Verification items for the finished model (mm, model axes). A direction names the side the tool comes from. Give positions to 0.01 mm unless a question says otherwise; leave off trailing zeros. Loops run counter-clockwise (first coordinate to the right, second up) from the corner with the lowest first, then second, coordinate; pieces in that order, holes last. Notation, with made-up numbers: M 23.25,35.25 L 37.25,35.25 A34 cw 37.25,70.25 Z; hole C -7.5,27.5 d2. An arc over 180 degrees is marked long. Use CSV: the item, a comma, the result in double quotes.
from build123d import *

# Parameters (mm, degrees)
F0_W        = 30
F0_H        = 5
F1_DEPTH    = 2
F2_R        = 5
F3_T1_DEPTH = 27


# Not quite as in the source:
# - a fillet or chamfer that OpenCascade refuses, or shapes differently, is made with other operations: its cross-section is extruded or revolved along the edge and cut away or added
# - a feature names something its author has since deleted; it is built from what else it names


with BuildPart() as f1:
    # F0 (on Top) → F1 (new body)
    with BuildSketch(Plane.XY):
        Polygon((0, 15), (0, 10), (30, 10), (30, 15), (8, 15), (4, 15), align=None)
        with Locations((15, 2.5)):
            Rectangle(F0_W, F0_H)
        with BuildLine():
            Line((0, 7.5), (0, 5))
            Line((0, 5), (30, 5))
            Line((30, 5), (30, 7.5))
            Line((30, 7.5), (24, 7.5))
            ThreePointArc((24, 7.5), (22.5, 6), (21, 7.5))
            Line((21, 7.5), (15, 7.5))
            Line((15, 7.5), (9, 7.5))
            ThreePointArc((9, 7.5), (7.5, 6), (6, 7.5))
            Line((6, 7.5), (0, 7.5))
        make_face()
        with BuildLine():
            Line((0, 10), (0, 7.5))
            Line((0, 7.5), (6, 7.5))
            ThreePointArc((6, 7.5), (7.5, 9), (9, 7.5))
            Line((9, 7.5), (15, 7.5))
            Line((15, 7.5), (21, 7.5))
            ThreePointArc((21, 7.5), (22.5, 9), (24, 7.5))
            Line((24, 7.5), (30, 7.5))
            Line((30, 7.5), (30, 10))
            Line((30, 10), (0, 10))
        make_face()
        Polygon((0, 60), (0, 15), (4, 15), (8, 15), (8, 60), align=None)
        Polygon((5, 25), (4, 25), (3, 25), (3, 55), (5, 55), align=None, mode=Mode.SUBTRACT)
    extrude(amount=F1_DEPTH)

    # F2
    f2_edges = [f1.edges().sort_by_distance(p)[0] for p in [
        (8, 15, 1),
        (30, 15, 1),
        (30, 0, 1),
        (0, 0, 1),
    ]]
    fillet(f2_edges, radius=F2_R)

    # F3: fillet of radius 5 on 2 edges, made by hand

    # F3_s2 → F3_t1 (cut)
    with BuildSketch(Plane.XY.offset(-12.5)):
        with BuildLine():
            ThreePointArc((3, 60), (6.5355339059, 58.5355339059), (8, 55))
            Line((8, 55), (8, 60))
            Line((8, 60), (3, 60))
        make_face()
        with BuildLine():
            ThreePointArc((0, 55), (1.4644660941, 58.5355339059), (5, 60))
            Line((5, 60), (0, 60))
            Line((0, 60), (0, 55))
        make_face()
    extrude(amount=F3_T1_DEPTH, mode=Mode.SUBTRACT)


solid = f1.part
(1) Section check A-A on x = 22.5. Record the cut outline in (y, z), plus the area to 3 significant figures.
Calculated:
outline,"M 0,0 L 6,0 L 6,2 L 0,2 Z; M 9,0 L 15,0 L 15,2 L 9,2 Z"
area,"24.0 mm²"
(2) Section check B-B on y = 7.5. Record the cut outline in (x, z).
Calculated:
outline,"M 0,0 L 6,0 L 6,2 L 0,2 Z; M 9,0 L 21,0 L 21,2 L 9,2 Z; M 24,0 L 30,0 L 30,2 L 24,2 Z"
(3) Section check D-D on z = 1.6. Record the cut outline in (x, y), plus the area to 3 significant figures.
Calculated:
outline,"M 0,5 A5 ccw 5,0 L 25,0 A5 ccw 30,5 L 30,10 A5 ccw 25,15 L 13,15 A5 cw 8,20 L 8,55 A5 ccw 4,59.9 A5 ccw 0,55 Z; hole M 3,25 L 5,25 L 5,55 L 3,55 Z; hole C 7.5,7.5 d3; hole C 22.5,7.5 d3"
area,"714 mm²"
(4) Depth check by flat-ended pin: pin 1 Ø1 at (x, z) = (22.5, 1.5) entering from +Y; pin 2 Ø0.6 at (y, z) = (30, 0.5) entering from +X. Enter the tip coordinate at first touch or a pass-through.
Calculated:
pin 1,"stops at y = 15"
pin 2,"stops at x = 8"
(5) Tool access check on faces 1 (the flat face through (4, 55, 1)), 2 (the flat face through (15, 0, 1)), 3 (the flat face through (8, 37, 1)). Record the directions out of +Z, -Z, +X, -X, +Y, -Y that give a thin tool (end or side, any length) a straight path to the whole face; none if there is none.
Calculated:
face 1,"+Z, -Z"
face 2,"+Z, -Z, +X, -X, -Y"
face 3,"+Z, -Z, +X, +Y"
(6) Scan lines: L1, parallel to X at y = 7.5, z = 0.5; L2, parallel to X at y = 35, z = 1.7; L3, parallel to Y at x = 22.5, z = 1.15. Record each from-to range of solid material in increasing order. Write a range as from..to.
Calculated:
L1,"x = 0..6, 9..21, 24..30"
L2,"x = 0..3, 5..8"
L3,"y = 0..6, 9..15"
(7) Section check C-C on y = 44.5. Record the cut outline in (x, z), plus the area to 3 significant figures.
Calculated:
outline,"M 0,0 L 3,0 L 3,2 L 0,2 Z; M 5,0 L 8,0 L 8,2 L 5,2 Z"
area,"12.0 mm²"
(8) Mould release check, pull along X, two halves, no side actions. Record for faces 4 (the flat face through (3, 40, 1)), 5 (the cylindrical face through (29, 13, 1)), 6 (the flat face through (0, 30, 1)): released by +X, released by -X, zero draft, split by the parting line, or undercut.
Calculated:
face 4,"undercut"
face 5,"released by +X"
face 6,"released by -X"
